Here's how the part is built. I have some questions about the finished solid (model axes, mm). A direction names the side the tool comes from. Coordinates: 2 decimals unless noted, no trailing zeros. Write each loop counter-clockwise with the first axis right and the second up, starting at its lowest first coordinate (ties: lowest second). Pieces come first, ordered by that corner, then holes. Notation, with made-up numbers: (60.25, 19.5) - (88.25, 19.5) arc R20 cw to (88.25, 34.5) - close; hole circle Ø11 at (77.25, 69.5). An arc over 180 degrees is marked (long way). Answer in a Markdown table with one row per item. Add a question column.
Item 1: Which directions (+Z, -Z, +X, -X, +Y, -Y) give clear straight access to the entire face, cutting with the end or side of a thin tool? Please do faces 4 (the face through (-1.565, 41.278, -3.035)), 5 (the face through (0, 49, -3)), 6 (the face through (13, 0, -3)), 7 (the face through (10.979, 20.826, 0.517)).
Item 2: We'd pull the mould along X, two halves only. Please class faces 1 (the face through (25.4, 19, -3)), 2 (the face through (13, 10, -18.542)), 3 (the face through (13, 38.1, -3)): +X half, -X half, draft (parallel to the pull), parting line (faces both ways), or undercut.
Item 3: If I drill on probe 1 along Y at (x, z) = (12.7, 10); probe 2 along Y at (x, z) = (14, 9); probe 3 along Z at (x, y) = (-0.9, -6.35), over which ranges is the centre line in solid material (lowest first)? Write a range as from..to.
Item 4: I'm going to push flat-ended pins straight in: pin 1 (10 mm diameter, centred on y = -6.35, z = -3.175, fed in from -X) (3 decimals); pin 2 (7.5 mm diameter, centred on x = 10, z = -10, fed in from +Y); pin 3 (12.5 mm diameter, centred on x = 12.7, y = 9.525, fed in from +Z); pin 4 (12.5 mm diameter, centred on x = 10.5, z = -14, fed in from -Y). Where does each tip first touch, or does it pass through?
Item 5: Imagine slicing it at A-A (y = -6.35). Please give me the cut outline in (x, z) (3 decimals), plus the area to 3 significant figures.
Item 6: Imagine slicing it at D-D (x = 12.7). Please give me the cut outline in (y, z).
Item 7: Imagine slicing it at B-B (x = -1.5). Please give me the cut outline in (y, z) (3 decimals), plus the area to 3 significant figures.
Item 8: Imagine slicing it at C-C (z = -2.5). Please give me the cut outline in (x, y) (1 decimal), plus the area to 3 significant figures.
from build123d import *

# Parameters (mm, degrees)
F0_W     = 38.1
F0_H     = 19.05
F1_DEPTH = 25.4
F3_DEPTH = 25.4
F2_R     = 7.9375
F4_DEPTH = 37.592
F5_W     = 12.7
F5_H     = 44.45
F5_W_2   = 38.1
F6_DEPTH = 3.175
F8_R     = 3.175
F7_R     = 3.175
F9_DEPTH = 25.4


with BuildPart() as f1:
    # F0 (on Right) → F1 (new body)
    with BuildSketch(Plane.YZ):
        with Locations((19.05, 9.525)):
            Rectangle(F0_W, F0_H)
    extrude(amount=F1_DEPTH)

    # F3 (add): a face of the model
    f3_faces = [f1.faces().sort_by_distance(p)[0] for p in [
        (12.7, 19.05, 0),
    ]]
    extrude(f3_faces, amount=F3_DEPTH)

    # F2 (on face) → F4 (cut)
    with BuildSketch(Plane.XY.offset(19.05)):
        with Locations((12.7, 28.575)):
            Circle(F2_R)
        with Locations((12.7, 9.525)):
            Circle(F2_R)
    extrude(amount=-F4_DEPTH, mode=Mode.SUBTRACT)

    # F5 (on face) → F6 (join)
    with BuildSketch(Plane(origin=(0, 0, 0), x_dir=(0, -1, 0), z_dir=(-1, 0, 0))):
        with Locations((-44.45, -3.175)):
            Rectangle(F5_W, F5_H)
        with Locations((-19.05, -3.175)):
            Rectangle(F5_W_2, F5_H)
        with Locations((6.35, -3.175)):
            Rectangle(F5_W, F5_H)
    extrude(amount=F6_DEPTH)

    # F8 (on face) + F7 (on face) → F9 (cut)
    with BuildSketch(Plane.YZ):
        with Locations((-6.35, -3.175)):
            Circle(F8_R)
    with BuildSketch(Plane.YZ):
        with Locations((44.45, -3.175)):
            Circle(F7_R)
    extrude(amount=-F9_DEPTH, mode=Mode.SUBTRACT)


solid = f1.part
Here are the results:
| question | item | result |
|---|---|---|
| 1 | face 4 | +X, -X |
| 1 | face 5 | +Z, -Z, +X, +Y |
| 1 | face 6 | +Z, -Z, +X, -Y |
| 1 | face 7 | +Z |
| 2 | face 1 | +X half |
| 2 | face 2 | undercut |
| 2 | face 3 | draft |
| 3 | probe 1 | y = 0..1.59, 17.46..20.64, 36.51..38.1 |
| 3 | probe 2 | y = 0..1.69, 17.36..20.74, 36.41..38.1 |
| 3 | probe 3 | z = -25.4..-6.35, 0..19.05 |
| 4 | pin 1 | stops at x = -3.175 |
| 4 | pin 2 | stops at y = 38.1 |
| 4 | pin 3 | stops at z = -18.54 |
| 4 | pin 4 | stops at y = 0 |
| 5 | outline | (-3.175, -25.4) - (0, -25.4) - (0, -6.35) - (-3.175, -6.35) - close; (-3.175, 0) - (0, 0) - (0, 19.05) - (-3.175, 19.05) - close |
| 5 | area | 121 mm2 |
| 6 | outline | (0, -25.4) - (38.1, -25.4) - (38.1, 19.05) - (36.51, 19.05) - (36.51, -18.54) - (20.64, -18.54) - (20.64, 19.05) - (17.46, 19.05) - (17.46, -18.54) - (1.59, -18.54) - (1.59, 19.05) - (0, 19.05) - close |
| 7 | outline | (-12.7, -25.4) - (50.8, -25.4) - (50.8, 19.05) - (-12.7, 19.05) - close; hole circle Ø6.35 at (-6.35, -3.175); hole circle Ø6.35 at (44.45, -3.175) |
| 7 | area | 2,760 mm2 |
| 8 | outline | (-3.2, -12.7) - (0, -12.7) - (0, -9.5) - (-3.2, -9.5) - close; (-3.2, -3.2) - (0, -3.2) - (0, 0) - (25.4, 0) - (25.4, 38.1) - (0, 38.1) - (0, 41.3) - (-3.2, 41.3) - close; (-3.2, 47.6) - (0, 47.6) - (0, 50.8) - (-3.2, 50.8) - close; hole circle Ø15.9 at (12.7, 9.5); hole circle Ø15.9 at (12.7, 28.6) |
| 8 | area | 734 mm2 |
